Autodesk Inventor part; units mm, degrees
ref_plane "YZ Plane" through (0, 0, 0) normal (1, 0, 0) x (0, 1, 0)
ref_plane "XZ Plane" through (0, 0, 0) normal (0, 1, 0) x (-1, 0, 0)
ref_plane "XY Plane" through (0, 0, 0) normal (0, 0, 1) x (1, 0, 0)
sketch "Sketch1" plane through (0, 0, 0) normal (1, 0, 0) x (0, 1, 0)
  circle A0 centre (-3.2893, 9.9949) radius 2.1463
  line L0 (2.2183, 3.2343) -> (-0.0365, 5.4891)
  arc A1 (1.6256, 1.8034) -> (2.2183, 3.2343) centre (1.6256, 2.6416) ccw
  line L1 (-0.4826, 1.8034) -> (1.6256, 1.8034)
  arc A2 (-0.4826, 1.8034) -> (-0.7874, 1.4986) centre (-0.4826, 1.4986) ccw
  line L2 (-0.7874, 0.7874) -> (-0.7874, 1.4986)
  arc A3 (-0.7874, 0.7874) -> (0, 0) centre (0, 0.7874) ccw
  line L3 (4.699, 0) -> (0, 0)
  arc A4 (4.699, 0) -> (6.7056, 2.0066) centre (4.699, 2.0066) ccw
  line L4 (6.7056, 6.7056) -> (6.7056, 2.0066)
  arc A5 (6.7056, 6.7056) -> (5.9182, 7.493) centre (5.9182, 6.7056) ccw
  line L5 (5.207, 7.493) -> (5.9182, 7.493)
  arc A6 (5.207, 7.493) -> (4.9022, 7.1882) centre (5.207, 7.1882) ccw
  line L6 (4.9022, 5.08) -> (4.9022, 7.1882)
  arc A7 (3.4713, 4.4873) -> (4.9022, 5.08) centre (4.064, 5.08) ccw
  line L7 (1.2165, 6.7421) -> (3.4713, 4.4873)
  arc A8 (0.3386, 8.8615) -> (1.2165, 6.7421) centre (3.3358, 8.8615) ccw
  line L8 (0.3386, 11.1283) -> (0.3386, 8.8615)
  arc A9 (1.2165, 13.2477) -> (0.3386, 11.1283) centre (3.3358, 11.1283) ccw
  line L9 (3.4713, 15.5025) -> (1.2165, 13.2477)
  arc A10 (4.9022, 14.9098) -> (3.4713, 15.5025) centre (4.064, 14.9098) ccw
  line L10 (4.9022, 12.8016) -> (4.9022, 14.9098)
  arc A11 (4.9022, 12.8016) -> (5.207, 12.4968) centre (5.207, 12.8016) ccw
  line L11 (5.9182, 12.4968) -> (5.207, 12.4968)
  arc A12 (5.9182, 12.4968) -> (6.7056, 13.2842) centre (5.9182, 13.2842) ccw
  line L12 (6.7056, 17.9832) -> (6.7056, 13.2842)
  arc A13 (6.7056, 17.9832) -> (4.699, 19.9898) centre (4.699, 17.9832) ccw
  line L13 (0, 19.9898) -> (4.699, 19.9898)
  arc A14 (0, 19.9898) -> (-0.7874, 19.2024) centre (0, 19.2024) ccw
  line L14 (-0.7874, 18.4912) -> (-0.7874, 19.2024)
  arc A15 (-0.7874, 18.4912) -> (-0.4826, 18.1864) centre (-0.4826, 18.4912) ccw
  line L15 (1.6256, 18.1864) -> (-0.4826, 18.1864)
  arc A16 (2.2183, 16.7555) -> (1.6256, 18.1864) centre (1.6256, 17.3482) ccw
  line L16 (-0.0365, 14.5007) -> (2.2183, 16.7555)
  arc A17 (-2.1559, 13.6228) -> (-0.0365, 14.5007) centre (-2.1559, 16.62) ccw
  line L17 (-4.4227, 13.6228) -> (-2.1559, 13.6228)
  arc A18 (-6.5421, 14.5007) -> (-4.4227, 13.6228) centre (-4.4227, 16.62) ccw
  line L18 (-8.7969, 16.7555) -> (-6.5421, 14.5007)
  arc A19 (-8.2042, 18.1864) -> (-8.7969, 16.7555) centre (-8.2042, 17.3482) ccw
  line L19 (-6.096, 18.1864) -> (-8.2042, 18.1864)
  arc A20 (-6.096, 18.1864) -> (-5.7912, 18.4912) centre (-6.096, 18.4912) ccw
  line L20 (-5.7912, 19.2024) -> (-5.7912, 18.4912)
  arc A21 (-5.7912, 19.2024) -> (-6.5786, 19.9898) centre (-6.5786, 19.2024) ccw
  line L21 (-11.2776, 19.9898) -> (-6.5786, 19.9898)
  arc A22 (-11.2776, 19.9898) -> (-13.2842, 17.9832) centre (-11.2776, 17.9832) ccw
  line L22 (-13.2842, 13.2842) -> (-13.2842, 17.9832)
  arc A23 (-13.2842, 13.2842) -> (-12.4968, 12.4968) centre (-12.4968, 13.2842) ccw
  line L23 (-11.7856, 12.4968) -> (-12.4968, 12.4968)
  arc A24 (-11.7856, 12.4968) -> (-11.4808, 12.8016) centre (-11.7856, 12.8016) ccw
  line L24 (-11.4808, 14.9098) -> (-11.4808, 12.8016)
  arc A25 (-10.0499, 15.5025) -> (-11.4808, 14.9098) centre (-10.6426, 14.9098) ccw
  line L25 (-7.7951, 13.2477) -> (-10.0499, 15.5025)
  arc A26 (-6.9172, 11.1283) -> (-7.7951, 13.2477) centre (-9.9144, 11.1283) ccw
  line L26 (-6.9172, 8.8615) -> (-6.9172, 11.1283)
  arc A27 (-7.7951, 6.7421) -> (-6.9172, 8.8615) centre (-9.9144, 8.8615) ccw
  line L27 (-10.0499, 4.4873) -> (-7.7951, 6.7421)
  arc A28 (-11.4808, 5.08) -> (-10.0499, 4.4873) centre (-10.6426, 5.08) ccw
  line L28 (-11.4808, 7.1882) -> (-11.4808, 5.08)
  arc A29 (-11.4808, 7.1882) -> (-11.7856, 7.493) centre (-11.7856, 7.1882) ccw
  line L29 (-12.4968, 7.493) -> (-11.7856, 7.493)
  arc A30 (-12.4968, 7.493) -> (-13.2842, 6.7056) centre (-12.4968, 6.7056) ccw
  line L30 (-13.2842, 2.0066) -> (-13.2842, 6.7056)
  arc A31 (-13.2842, 2.0066) -> (-11.2776, 0) centre (-11.2776, 2.0066) ccw
  line L31 (-6.5786, 0) -> (-11.2776, 0)
  arc A32 (-6.5786, 0) -> (-5.7912, 0.7874) centre (-6.5786, 0.7874) ccw
  line L32 (-5.7912, 1.4986) -> (-5.7912, 0.7874)
  arc A33 (-5.7912, 1.4986) -> (-6.096, 1.8034) centre (-6.096, 1.4986) ccw
  line L33 (-8.2042, 1.8034) -> (-6.096, 1.8034)
  arc A34 (-8.7969, 3.2343) -> (-8.2042, 1.8034) centre (-8.2042, 2.6416) ccw
  line L34 (-6.5421, 5.4891) -> (-8.7969, 3.2343)
  arc A35 (-4.4227, 6.367) -> (-6.5421, 5.4891) centre (-4.4227, 3.3698) ccw
  line L35 (-2.1559, 6.367) -> (-4.4227, 6.367)
  arc A36 (-0.0365, 5.4891) -> (-2.1559, 6.367) centre (-2.1559, 3.3698) ccw
extrude "Extrusion1" add sketch "Sketch1" along normal blind 25.4
properties part number "Extruson profile"
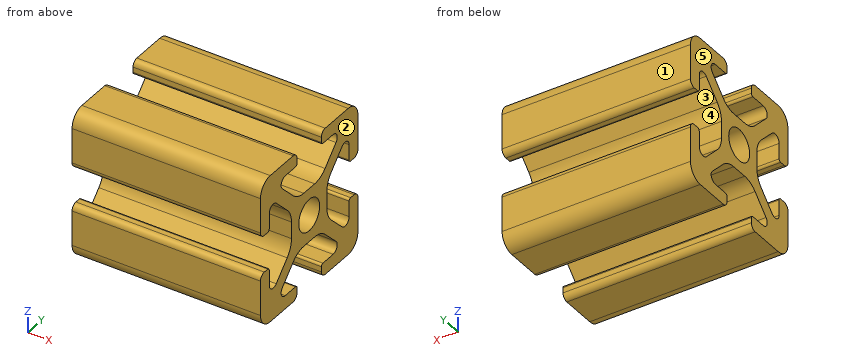
Read the model definition and answer for the solid it produces. Units are mm, in the model's axes. Face numbers are marked on the shaded views. A direction names the side the tool comes from. Round coordinates to 2 decimals unless told otherwise and drop trailing zeros. Write each loop counter-clockwise with the first axis right and the second up, starting at its lowest first coordinate (ties: lowest second). Pieces come first, ordered by that corner, then holes. Notation, with made-up numbers: (37.25, -24) - (72.25, -24) arc R31 ccw to (72.25, 9) - close; hole circle Ø6 at (-36.5, 40). An arc over 180 degrees is marked (long way). One line per item, written item: value.
Q1. Find section B-B (y = -7.25). Determine the outline of the cut face in (x, z), and give its area (3 significant figures).
The answers:
outline: (0, 0) - (25.4, 0) - (25.4, 1.8) - (0, 1.8) - close; (0, 4.78) - (25.4, 4.78) - (25.4, 7.49) - (0, 7.49) - close; (0, 12.5) - (25.4, 12.5) - (25.4, 15.21) - (0, 15.21) - close; (0, 18.19) - (25.4, 18.19) - (25.4, 19.99) - (0, 19.99) - close
area: 229 mm2
Q2. Straight lines are drawn through the part: line 1 (Y direction, x = 10.5, z = 14.5); line 2 (Z direction, x = 7.5, y = -10.75); line 3 (Y direction, x = 13.25, z = 7). For each, find the intervals that lie inside material, in ascending order. Write a range as from..to.
The answers:
line 1: y = -13.28..-11.48, -9.05..-6.54, -0.04..2.47, 4.9..6.71
line 2: z = 0..4.25, 15.74..19.99
line 3: y = -13.23..-11.48, -7.57..0.99, 4.9..6.65
Q3. Each of these flat-tipped pins is pushed along its axis until it touches: P1, Ø0.6, axis at x = 15.5, z = 18.5, coming from the -Y side; P2, Ø2.5, axis at x = 10.5, y = -3, coming from the -Z side; P3, Ø4, axis at y = -3.29, z = 9.99, coming from the -X side; P4, Ø1.1, axis at x = 6.5, y = -3.5, coming from the +Z side. Where does it stop, or does it pass through?
The answers:
P1: stops at y = -13.27
P2: stops at z = 6.34
P3: passes through
P4: stops at z = 13.62
Q4. Find section A-A (z = 11.5). Determine the outline of the cut face in (x, y), and give its area (3 significant figures).
The answers:
outline: (0, -6.94) - (25.4, -6.94) - (25.4, -4.82) - (0, -4.82) - close; (0, -1.76) - (25.4, -1.76) - (25.4, 0.36) - (0, 0.36) - close
area: 108 mm2
Q5. Which of the six approach directions +Z, -Z, +X, -X, +Y, -Y give full straight-line access (tool end or side, diameter ignored) to the marked faces 4 and 5?
The answers:
face 4: +X, -X
face 5: +Z, -Z, -X, +Y, -Y
Q6. For a pull along Y with two mould halves and no side action, classify the marked faces 1, 2 and 3 as pulls with the +Y half, pulls with the -Y half, needs draft (parallel to the pull), parting line crosses it, or undercut.
The answers:
face 1: pulls with the +Y half
face 2: needs draft
face 3: undercut
Q7. Find section C-C (y = -9.5). Determine the outline of the cut face in (x, z).
The answers:
outline: (0, 0) - (25.4, 0) - (25.4, 5.04) - (0, 5.04) - close; (0, 14.95) - (25.4, 14.95) - (25.4, 19.99) - (0, 19.99) - close
